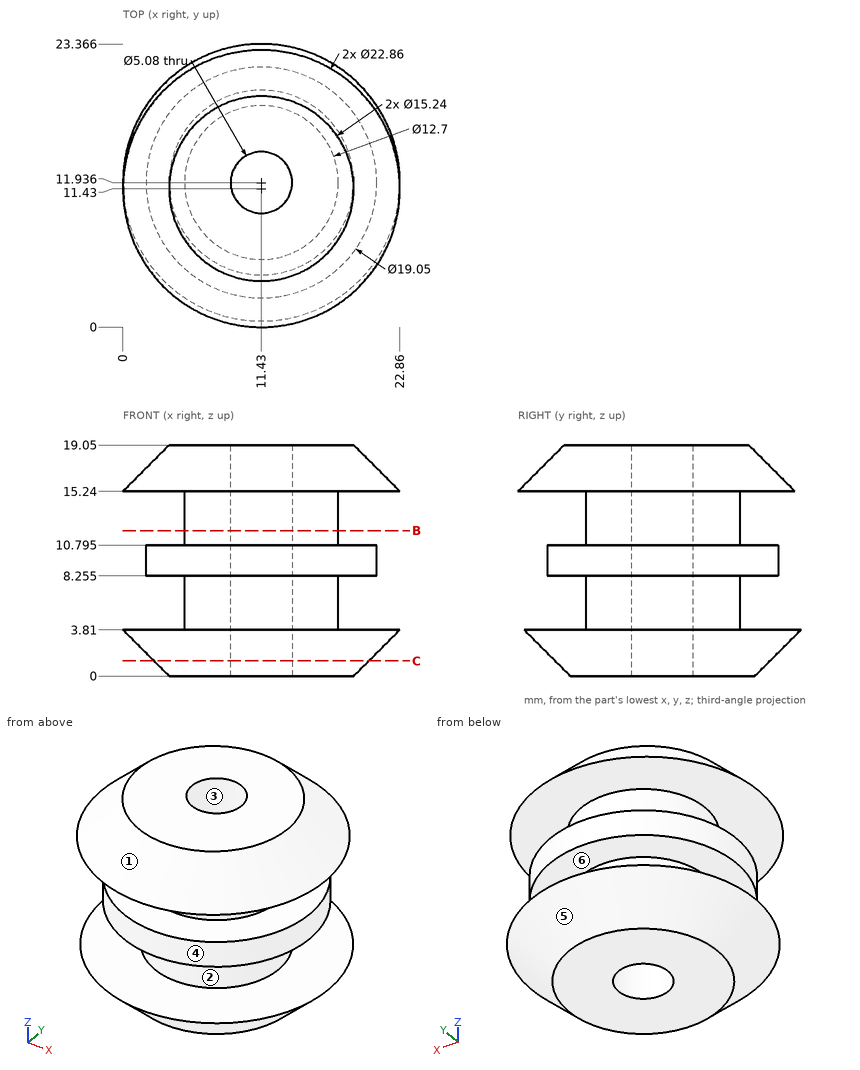
Print and shaded views of the part. All mm, measured from the part's lowest x, y and z. A direction names the side the tool comes from. Round coordinates to 2 decimals unless told otherwise and drop trailing zeros. Write each loop counter-clockwise with the first axis right and the second up, starting at its lowest first coordinate (ties: lowest second). Pieces come first, ordered by that corner, then holes.
Item 1: Cut at B-B, the plane z = 12. Give the cut face in (x, y), plus the area to 3 significant figures.
Results:
outline: circle Ø12.7 at (11.43, 11.94); hole circle Ø5.08 at (11.43, 11.94)
area: 106 mm2
Item 2: Probe L1, parallel to Y at x = 11.43, z = 14.5; L2, parallel to Y at x = 11.43, z = 8.5; L3, parallel to Z at x = 2, y = 8.75 (1 decimal). List the from-to ranges inside material, lowest first.
Results:
L1: y = 5.59 to 9.4, 14.48 to 18.29
L2: y = 2.41 to 9.4, 14.48 to 21.46
L3: z = 2.3 to 3.8, 15.2 to 16.9
Item 3: Two-plate mould, pull along Z, no slides. Class the marked faces 1, 2, 3 and 4: +Z half, -Z half, draft (parallel to the pull), parting line (faces both ways), or undercut.
Results:
face 1: +Z half
face 2: undercut
face 3: draft
face 4: undercut
Item 4: Drop flat-ended pins along their axis: pin 1 Ø1.5 at (x, y) = (15.5, 4) entering from -Z; pin 2 Ø9.5 at (x, y) = (10, 15.5) entering from -Z; pin 3 Ø2 at (x, z) = (10, 4) entering from -Y (1 decimal); pin 4 Ø1 at (x, z) = (10.5, 4) entering from +Y. Give the stop position or say it passes through.
Results:
pin 1: stops at z = 0.55
pin 2: stops at z = 0
pin 3: stops at y = 0.5
pin 4: stops at y = 23.36
Item 5: Which spindle directions (+Z, -Z, +X, -X, +Y, -Y) get a long thin tool onto all of the face, cutting with end or side? Do the marked faces 5 and 6. Say none if no direction does.
Results:
face 5: -Z
face 6: none
Item 6: Cut at C-C, the plane z = 1.25. Give the cut face in (x, y).
Results:
outline: circle Ø17.74 at (11.43, 11.94); hole circle Ø5.08 at (11.43, 11.94)
